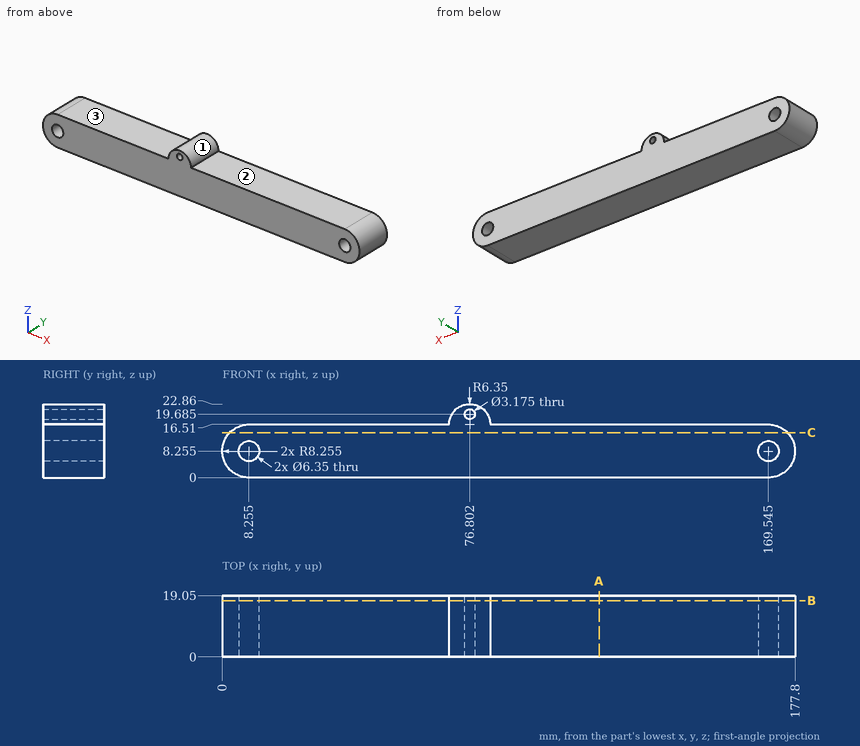
Here's the drawing with two shaded views (mm, measured from the low corner). I have some questions. A direction names the side the tool comes from. Round coordinates to 2 decimals unless told otherwise and drop trailing zeros. Loops run counter-clockwise (first coordinate to the right, second up) from the corner with the lowest first, then second, coordinate; pieces in that order, holes last. Notation, with made-up numbers: M 60.25,14.5 L 87.25,14.5 A23 ccw 87.25,26.5 Z; hole C 2,-7.5 d4. An arc over 180 degrees is marked long. Answer as a JSON object with one key per item and string values. Group by question number.
Q1. Will these pins go through, and if not, where does the flat tip stop? pin 1 (10 mm diameter, centred on x = 46, y = 12, fed in from +Z); pin 2 (4 mm diameter, centred on y = 3, z = 14, fed in from -X).
Q2. Imagine slicing it at A-A, the plane x = 117. Please give me the cut outline in (y, z).
Q3. Please list where these lines run through material, in increasing order: L1, parallel to X at y = 10.25, z = 10 (1 decimal); L2, parallel to X at y = 14.5, z = 6.75; L3, parallel to Z at x = 141.5, y = 16.5.
Q4. Imagine slicing it at B-B, the plane y = 17.5. Count the separate pieces of the cut face and the enclosed holes in it, then the cut area to 3 significant figures.
Q5. Imagine slicing it at C-C, the plane z = 14. Please give me the cut outline in (x, y), then the cut area to 3 significant figures.
Q6. On a 3-axis mill with a long thin cutter (end or side, diameter ignored), from which of +Z, -Z, +X, -X, +Y, -Y can I reach the whole of each face in a straight line? I mean the marked faces 1, 2 and 3. Say none if no direction works.
Findings:
{
 "1": {"pin 1": "stops at z = 16.51", "pin 2": "stops at x = 0.9"},
 "2": {"outline": "M 0,0 L 19.05,0 L 19.05,16.51 L 0,16.51 Z"},
 "3": {"L1": "x = 0.2 to 5.6, 10.9 to 166.9, 172.2 to 177.6", "L2": "x = 0.14 to 5.46, 11.05 to 166.75, 172.34 to 177.66", "L3": "z = 0 to 16.51"},
 "4": {"separate pieces": "1", "enclosed holes": "3", "area": "2,870 mm2"},
 "5": {"outline": "M 2.33,0 L 175.47,0 L 175.47,19.05 L 2.33,19.05 Z", "area": "3,300 mm2"},
 "6": {"face 1": "+Z, +Y, -Y", "face 2": "+Z, +X, +Y, -Y", "face 3": "+Z, -X, +Y, -Y"}
}
